Autodesk Inventor part; units mm, degrees
ref_plane "Work Plane2" through (-3, 86.25, 0) normal (0, 1, 0) x (1, 0, 0)
ref_plane "YZ Plane" through (0, 0, 0) normal (1, 0, 0) x (0, 1, 0)
ref_plane "XZ Plane" through (0, 0, 0) normal (0, 1, 0) x (-1, 0, 0)
sketch "Sketch1" plane through (0, 0, 0) normal (0, 0, 1) x (1, 0, 0)
  line L0 (0, 0) -> (20, 0)
  line L1 (20, 0) -> (20, 172.5)
  line L2 (20, 172.5) -> (0, 172.5)
  line L3 (0, 172.5) -> (0, 0)
  line L4 (0, 0) -> (0, 172.5)
  line L5 (0, 172.5) -> (-3, 172.5)
  line L6 (-3, 172.5) -> (-3, 0)
  line L7 (-3, 0) -> (0, 0)
  line L8 (20, 172.5) -> (20, 0)
  line L9 (20, 0) -> (23, 0)
  line L10 (23, 0) -> (23, 172.5)
  line L11 (23, 172.5) -> (20, 172.5)
  line L12 (23, 20) -> (-3, 20)
  point P0 (0, 20)
  point P1 (20, 20)
  dimension "d0" = 20
  dimension "d1" = 172.5
  dimension "d2" = 3
  dimension "d3" = 3
  dimension "d6" = 20
extrude "Extrusion1" add sketch "Sketch1" along normal blind 3
extrude "Extrusion2" add sketch "Sketch1" against normal blind 20 contours L7 L6 L12 L3 | L1 L12 L10 L9
chamfer "Chamfer1" distance 20 angle 35 1 edges at (-1.5, 20, -20) measured on face at (-1, 20, -6.6667)
chamfer "Chamfer2" distance 20 angle 35 1 edges at (21.5, 20, -20) measured on face at (22, 20, -6.6667)
sketch "Sketch2" plane through (0, 0, 3) normal (0, 0, 1) x (1, 0, 0)
  circle A0 centre (10, 162.6846) radius 2
  circle A1 centre (10, 142.6846) radius 2
  point P0 (0, 0)
extrude "Extrusion3" cut sketch "Sketch2" against normal through all
ref_plane "Work Plane2" through (-3, 86.25, 0) normal (0, 1, 0) x (1, 0, 0)
mirror "Mirror2" about plane through (-3, 86.25, 0) normal (0, 1, 0) of "Extrusion2", "Chamfer1", "Chamfer2"
fillet "Fillet1" radius 2 4 edges at (23, 0, -8.5) (-3, 0, -8.5) (23, 172.5, -8.5) (-3, 172.5, -8.5)
properties part number "Z Drill Template"
Model file for the job. Use its own axes, mm. A direction names the side the tool comes from. Round coordinates to 2 decimals unless told otherwise and drop trailing zeros. Order: outer loops, then holes, each group sorted by start corner. A loop starts at its lowest first (then second) coordinate and runs counter-clockwise, first axis right, second up. Notation, with made-up numbers: M 30,85.5 L 35,85.5 A30 cw 35,109.5 Z; hole C 21,83 d9. An arc over 180 degrees is marked long. Use CSV: the item, a comma, the result in double quotes.
Item 1: Saw through at D-D (y = 106). List the corners of the cut face in (x, z), plus the area to 3 significant figures.
Worked answers:
outline,"M -3,0 L 23,0 L 23,3 L -3,3 Z"
area,"78.0 mm²"
Item 2: Which spindle directions (+Z, -Z, +X, -X, +Y, -Y) get a long thin tool onto all of the face, cutting with end or side? Do faces 4 (the face through (20, 8, -8)), 5 (the face through (22, 169, -20)), 6 (the face through (22, 13, -10)), 7 (the face through (10, 87, 0)). Say none if no direction does.
Worked answers:
face 4,"-Z, +Y, -Y"
face 5,"-Z, +X, -X, +Y, -Y"
face 6,"-Z, +X, -X"
face 7,"-Z"
Item 3: Saw through at A-A (x = 10). List the corners of the cut face in (y, z).
Worked answers:
outline,"M 0,0 L 140.68,0 L 140.68,3 L 0,3 Z; M 144.68,0 L 160.68,0 L 160.68,3 L 144.68,3 Z; M 164.68,0 L 172.5,0 L 172.5,3 L 164.68,3 Z"
Item 4: Saw through at C-C (z = -16.75). List the corners of the cut face in (x, y).
Worked answers:
outline,"M -3,2 A2 ccw -1,0 L 0,0 L 0,8.27 L -3,8.27 Z; M -3,164.23 L 0,164.23 L 0,172.5 L -1,172.5 A2 ccw -3,170.5 Z; M 20,0 L 21,0 A2 ccw 23,2 L 23,8.27 L 20,8.27 Z; M 20,164.23 L 23,164.23 L 23,170.5 A2 ccw 21,172.5 L 20,172.5 Z"
Item 5: Pull direction X, two halves, no side cores. Call faces 1 (the face through (0, 165, -8)), 2 (the face through (23, 86, 1)), 3 (the face through (-1, 169, -20)): released by +X, released by -X, zero draft, split by the parting line, or undercut.
Worked answers:
face 1,"undercut"
face 2,"released by +X"
face 3,"zero draft"
Item 6: Probe probe 1 along Y at (x, z) = (10, 1.75); probe 2 along X at (y, z) = (154, -1); probe 3 along Z at (x, y) = (7.25, 54.5). List the from-to ranges inside material, lowest first.
Worked answers:
probe 1,"0 to 140.68, 144.68 to 160.68, 164.68 to 172.5"
probe 2,"-3 to 0, 20 to 23"
probe 3,"0 to 3"
Item 7: Pin check, flat tips, straight feed: pin 1 (4 mm diameter, centred on x = 19.5, y = 129.5, fed in from -Z); pin 2 (10 mm diameter, centred on y = 33.5, z = -6.5, fed in from -X). Stop position of each tip, or through.
Worked answers:
pin 1,"z = 0"
pin 2,"through"
Item 8: Saw through at B-B (z = -6.25). List the corners of the cut face in (x, y).
Worked answers:
outline,"M -3,2 A2 ccw -1,0 L 0,0 L 0,15.62 L -3,15.62 Z; M -3,156.88 L 0,156.88 L 0,172.5 L -1,172.5 A2 ccw -3,170.5 Z; M 20,0 L 21,0 A2 ccw 23,2 L 23,15.62 L 20,15.62 Z; M 20,156.88 L 23,156.88 L 23,170.5 A2 ccw 21,172.5 L 20,172.5 Z"
